Geometry: final body of the model. Coordinates: model frame, mm. A direction names the side the tool comes from. Give positions to 0.01 mm unless a question says otherwise; leave off trailing zeros. Write each loop counter-clockwise with the first axis right and the second up, starting at its lowest first coordinate (ties: lowest second). Pieces come first, ordered by that corner, then holes. Notation, with made-up numbers: (-3.75, -25) -> (10.25, -25) arc R13 ccw to (10.25, -21) -> close; hole circle Ø5 at (43.5, 24.25). An arc over 180 degrees is marked (long way). Answer as a JSON object with one key per item and string values.
from build123d import *

# Parameters (mm, degrees)
SKETCH1_R           = 9.525
BOSS_EXTRUDE1_DEPTH = 8.89
SKETCH2_R           = 3.175
BOSS_EXTRUDE2_DEPTH = 9.525
SKETCH3_R           = 2.38125
BOSS_EXTRUDE3_DEPTH = 8.89
CUT_EXTRUDE1_DEPTH  = 5.08


with BuildPart() as part:
    # Sketch1 → Boss-Extrude1 (new body)
    with BuildSketch(Plane.XY):
        Circle(SKETCH1_R)
    extrude(amount=-BOSS_EXTRUDE1_DEPTH)

    # Sketch2 → Boss-Extrude2 (add)
    with BuildSketch(Plane.XY):
        Circle(SKETCH2_R)
    extrude(amount=BOSS_EXTRUDE2_DEPTH)

    # Sketch3 → Boss-Extrude3 (add)
    with BuildSketch(Plane.XY.offset(9.525)):
        Circle(SKETCH3_R)
    extrude(amount=BOSS_EXTRUDE3_DEPTH)

    # Sketch4 → Cut-Extrude1 (cut)
    with BuildSketch(Plane.XY.offset(18.415)):
        with BuildLine():
            Line((-4.269996199, 0.889), (4.269996199, 0.889))
            ThreePointArc((4.269996199, 0.889), (0, 5.158996199), (-4.269996199, 0.889))
        make_face()
    extrude(amount=-CUT_EXTRUDE1_DEPTH, mode=Mode.SUBTRACT)


solid = part.part
Q1. Set-up query: faces 1 (the flat face through (0, 0, -8.89)), 2 (the flat face through (0, 1.5, 13.335)), 3 (the cylindrical face through (-0.69, -3.1, 4.7)). Return all of +Z, -Z, +X, -X, +Y, -Y with unobstructed straight access to the full face (end or side cutting, diameter ignored); none if empty.
Values:
{"face 1": "-Z, +X, -X, +Y, -Y", "face 2": "+Z, +X, -X, +Y", "face 3": "+Z"}
Q2. First-contact query: P1, Ø0.7, axis at x = -1, y = 1.5, coming from the +Z side (3 decimals); P2, Ø5, axis at x = 4.5, y = -4, coming from the +Z side; P3, Ø2, axis at x = -0.5, z = 15.5, coming from the +Y side. Flat tips, straight axial feed; report the tip coordinate or a pass-through.
Values:
{"P1": "z = 13.335", "P2": "z = 0", "P3": "y = 0.89"}
Q3. Cut plane D-D (x = 6). Return the cut outline in (y, z), and give its area (3 significant figures).
Values:
{"outline": "(-7.4, -8.89) -> (7.4, -8.89) -> (7.4, 0) -> (-7.4, 0) -> close", "area": "132 mm²"}
Q4. Cut plane A-A (x = 0). Return the cut outline in (y, z) (3 decimals), and give its area (3 significant figures).
Values:
{"outline": "(-9.525, -8.89) -> (9.525, -8.89) -> (9.525, 0) -> (3.175, 0) -> (3.175, 9.525) -> (2.381, 9.525) -> (2.381, 13.335) -> (0.889, 13.335) -> (0.889, 18.415) -> (-2.381, 18.415) -> (-2.381, 9.525) -> (-3.175, 9.525) -> (-3.175, 0) -> (-9.525, 0) -> close", "area": "265 mm²"}
Q5. Cut plane B-B (y = 0). Return the cut outline in (x, z) (3 decimals), and give its area (3 significant figures).
Values:
{"outline": "(-9.525, -8.89) -> (9.525, -8.89) -> (9.525, 0) -> (3.175, 0) -> (3.175, 9.525) -> (2.381, 9.525) -> (2.381, 18.415) -> (-2.381, 18.415) -> (-2.381, 9.525) -> (-3.175, 9.525) -> (-3.175, 0) -> (-9.525, 0) -> close", "area": "272 mm²"}
Q6. Cut plane C-C (z = -1.75). Return the cut outline in (x, y) (3 decimals), and give its area (3 significant figures).
Values:
{"outline": "circle Ø19.05 at (0, 0)", "area": "285 mm²"}
Q7. Material intervals for L1, parallel to Z at x = -6.25, y = 3.75; L2, parallel to Y at x = 0, z = -7.25 (3 decimals); L3, parallel to Y at x = 0, z = 7.25 (3 decimals), sorted ascending. Write a range as from..to.
Values:
{"L1": "-8.89..0", "L2": "-9.525..9.525", "L3": "-3.175..3.175"}
